Geometry check sheet. Reference: the model listing, model coordinates, mm. A direction names the side the tool comes from. Give positions to 0.01 mm unless a question says otherwise; leave off trailing zeros. Loops run counter-clockwise (first coordinate to the right, second up) from the corner with the lowest first, then second, coordinate; pieces in that order, holes last. Notation, with made-up numbers: (81, 54) -> (95, 54) arc R15 cw to (95, 58) -> close; hole circle Ø11 at (8, -19.5). An arc over 180 degrees is marked (long way). One line per item, written item: value. Start each with the question number.
(1) Tool access check on faces 1 (the face through (1.03, 25.13, 1.34)), 2 (the face through (1.03, 41.37, 1.34)), 3 (the face through (0, 39, -3.15)). Record the directions out of +Z, -Z, +X, -X, +Y, -Y that give a thin tool (end or side, any length) a straight path to the whole face; none if there is none.
(2) Gauge pin test, flat end, axial feed: pin 1 Ø1.5 at (y, z) = (39, 1) entering from +X. Record the tip position at first contact, or that the pin passes through.
(3) Sectioned sample at C-C, the plane y = 17. Record the cut outline in (x, z).
(4) Scan lines: line 1 along Y through (x, z) = (-0.25, -2); line 2 along X through (y, z) = (29, 0.25). Record each from-to range of solid material in increasing order. Write a range as from..to.
from build123d import *

# Parameters (mm, degrees)
BOSS_EXTRUDE1_DEPTH = 2.7432


with BuildPart() as part:
    # Sketch1 → Revolve1 (revolve)
    with BuildSketch(Plane.XY, mode=Mode.PRIVATE) as revolve1_sk:
        Polygon((0, 0), (1.6764, 0), (1.6764, 12.7), (1.6891, 12.7), (1.6891, 37.211), (3.1115, 37.211), (3.1115, 39.9542), (1.6891, 39.9542), (1.6891, 42.7482), (1.6764, 42.7482), (1.6764, 47.1424), (0, 47.1424), align=None)
    revolve(revolve1_sk.sketch.rotate(Axis((0, 0, 0), (0, 1, 0)), 90), axis=Axis((0, 0, 0), (0, 1, 0)))  # turned: the seam where the file's is

    # Sketch2 → Boss-Extrude1 (add)
    with BuildSketch(Plane(origin=(0, 39.9542, 0), x_dir=(1, 0, 0), z_dir=(0, 1, 0))):
        Polygon((3.636844816, 0), (1.818422408, 3.1496), (-1.818422408, 3.1496), (-3.636844816, 0), (-1.818422408, -3.1496), (1.818422408, -3.1496), align=None)
    extrude(amount=-BOSS_EXTRUDE1_DEPTH)


solid = part.part
Calculated:
1. face 1: -Y
1. face 2: +Y
1. face 3: -Z, +X, -X, +Y, -Y
2. pin 1: stops at x = 3.49
3. outline: circle Ø3.38 at (0, 0)
4. line 1: y = 37.21..39.95
4. line 2: x = -1.67..1.67
